from build123d import *

# Parameters (mm, degrees)
F0_W     = 115
F0_H     = 120
F0_H_2   = 10
F1_DEPTH = 5
F2_DEPTH = 35
F3_DEPTH = 25
F4_DEPTH = 80


with BuildPart() as f1:
    # F0 (on Top) → F1 (new body)
    with BuildSketch(Plane.XY):
        with Locations((-57.5, -75)):
            Rectangle(F0_W, F0_H)
        Polygon((0, -5), (0, 0), (-115, 0), (-120, 0), (-120, -140), (-115, -140), (0, -140), (0, -135), (-115, -135), (-115, -15), (-115, -5), align=None)
        with Locations((-57.5, -10)):
            Rectangle(F0_W, F0_H_2)
    extrude(amount=-F1_DEPTH)

    # F0 (on Top) → F2 (join)
    with BuildSketch(Plane.XY):
        with Locations((-57.5, -10)):
            Rectangle(F0_W, F0_H_2)
        Polygon((0, -5), (0, 0), (-115, 0), (-120, 0), (-120, -140), (-115, -140), (0, -140), (0, -135), (-115, -135), (-115, -15), (-115, -5), align=None)
    extrude(amount=F2_DEPTH)

    # F0 (on Top) → F3 (cut)
    with BuildSketch(Plane.XY):
        with Locations((-57.5, -10)):
            Rectangle(F0_W, F0_H_2)
    extrude(amount=F3_DEPTH, mode=Mode.SUBTRACT)

    # F2_face (on face) → F4 (join)
    with BuildSketch(Plane(origin=(0, -64.782609, 6.413043), x_dir=(0, 1, 0), z_dir=(1, 0, 0))):
        Polygon((-75.217391, 28.586957), (-75.217391, -11.413043), (64.782609, -11.413043), (64.782609, 28.586957), (49.782609, 28.586957), (49.782609, 18.586957), (59.782609, 18.586957), (59.782609, -6.413043), (-70.217391, -6.413043), (-70.217391, 28.586957), align=None)
    extrude(amount=F4_DEPTH)


solid = f1.part
Input: part model. Units: mm. Frame: model coordinates. A direction names the side the tool comes from. Give positions to 0.01 mm unless a question says otherwise; leave off trailing zeros. Order: outer loops, then holes, each group sorted by start corner. A loop starts at its lowest first (then second) coordinate and runs counter-clockwise, first axis right, second up.
Q1. Section A-A on z = 28. Output: boundary loops of the cut face in (x, y), and give its area (3 significant figures).
Checked values:
outline: (-120, -140) - (80, -140) - (80, -135) - (-115, -135) - (-115, -15) - (80, -15) - (80, 0) - (-120, 0) - close
area: 4,600 mm2
Q2. Draft query along Y for faces 4 (the flat face through (-21, -140, 15)), 5 (the flat face through (-120, -69, 15)), 6 (the flat face through (-19, -5, 13)). Return one class per face: +Y half, -Y half, draft (parallel to the pull), parting line (faces both ways), or undercut.
Checked values:
face 4: -Y half
face 5: draft
face 6: undercut
Q3. Section C-C on x = -63.5. Output: boundary loops of the cut face in (y, z), and give its area (3 significant figures).
Checked values:
outline: (-140, -5) - (0, -5) - (0, 35) - (-15, 35) - (-15, 25) - (-5, 25) - (-5, 0) - (-135, 0) - (-135, 35) - (-140, 35) - close
area: 1,150 mm2
Q4. Set-up query: faces 1 (the flat face through (-43, -13, 35)), 2 (the flat face through (-19, -10, 25)), 3 (the flat face through (-19, -15, 30)). Return all of +Z, -Z, +X, -X, +Y, -Y with unobstructed straight access to the full face (end or side cutting, diameter ignored); none if empty.
Checked values:
face 1: +Z, +X, -X, +Y, -Y
face 2: +X
face 3: +Z, +X
Q5. Ray query, probe 1 along Y at (x, z) = (62, 20.5); probe 2 along Y at (x, z) = (-84, 26); probe 3 along Z at (x, y) = (-58, -9.5). Return the intervals inside material, ascending.
Checked values:
probe 1: y = -140 to -135, -5 to 0
probe 2: y = -140 to -135, -15 to 0
probe 3: z = -5 to 0, 25 to 35
Q6. Section B-B on y = -44. Output: boundary loops of the cut face in (x, z), and give its area (4 significant figures).
Checked values:
outline: (-120, -5) - (80, -5) - (80, 0) - (-115, 0) - (-115, 35) - (-120, 35) - close
area: 1,175 mm2
Q7. Section D-D on z = 17. Output: boundary loops of the cut face in (x, y).
Checked values:
outline: (-120, -140) - (80, -140) - (80, -135) - (-115, -135) - (-115, -5) - (80, -5) - (80, 0) - (-120, 0) - close
Q8. Contact query for flat-ended pins moving along their axis: pin 1 Ø10.5 at (y, z) = (-76.5, 18.5) entering from +X; pin 2 Ø4 at (x, y) = (30, -17.5) entering from +Z. Output: stop coordinate, or through.
Checked values:
pin 1: stops at x = -115
pin 2: stops at z = 0
